Input: dimensioned drawing with shaded views. Units: mm. Origin: part minimum x, y, z. A direction names the side the tool comes from. Give positions to 0.01 mm unless a question says otherwise; leave off trailing zeros. Write each loop counter-clockwise with the first axis right and the second up, starting at its lowest first coordinate (ties: lowest second). Pieces come first, ordered by that corner, then holes. Notation, with made-up numbers: (75.5, 79) -> (102.5, 79) arc R27 ccw to (102.5, 104) -> close; hole circle Ø3 at (-15, 86.5). An arc over 180 degrees is marked (long way). Return JSON: item names as keys, results as strings. Group by question number.
Item 1: Section D-D, the plane y = 19. Return loops of the section in (x, z), then the cut area to 3 significant figures.
Item 2: Set-up query: the marked faces 1, 2 and 3. Return all of +Z, -Z, +X, -X, +Y, -Y with unobstructed straight access to the full face (end or side cutting, diameter ignored); none if empty.
Item 3: Line query: line 1 (Y direction, x = 6, z = 2.4); line 2 (Y direction, x = 5.25, z = 1.35) (1 decimal); line 3 (X direction, y = 6, z = 2.2). Output: solid intervals per line, ascending. Write a range as [from, to].
Item 4: Mould query, pull axis X, two halves, no side actions, for the marked faces 4, 5 and 6. Classes: released by +X, released by -X, zero draft, split by the parting line, or undercut.
Item 5: Section B-B, the plane z = 0.9. Count the separate pieces of the cut face and the enclosed holes in it, then the cut area to 3 significant figures.
Item 6: Pin query (flat end, axial travel): P1, Ø5, axis at x = 5, y = 6.5, coming from the +Z side; P2, Ø2, axis at x = 6, y = 25, coming from the +Z side; P3, Ø3, axis at x = 10, z = 0.5, coming from the +Y side (1 decimal). Return the tip coordinate at first contact, or that it passes through.
Item 7: Section A-A, the plane y = 6. Return loops of the section in (x, z).
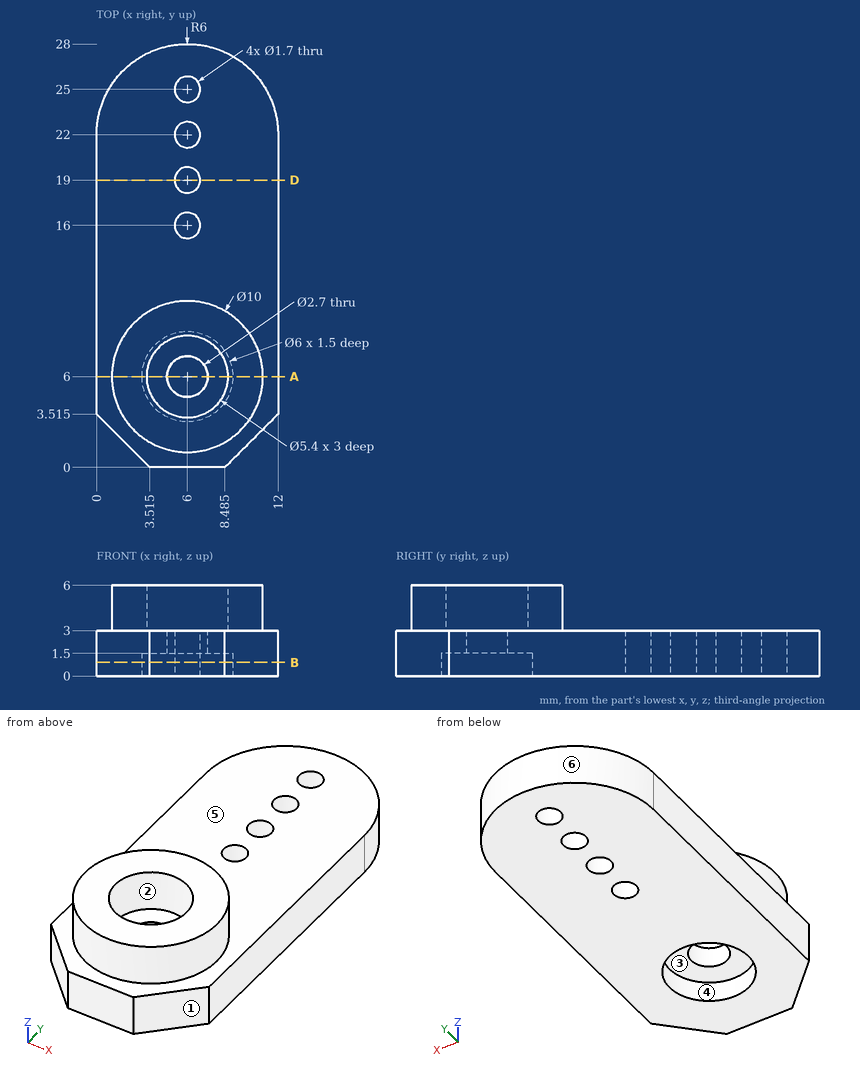
Answer below:
{
 "1": {"outline": "(0, 0) -> (5.15, 0) -> (5.15, 3) -> (0, 3) -> close; (6.85, 0) -> (12, 0) -> (12, 3) -> (6.85, 3) -> close", "area": "30.9 mm2"},
 "2": {"face 1": "+Z, -Z, +X, -Y", "face 2": "+Z", "face 3": "-Z"},
 "3": {"line 1": "y = [0, 4.65], [7.35, 15.15], [16.85, 18.15], [19.85, 21.15], [22.85, 24.15], [25.85, 28]", "line 2": "y = [0, 3.1], [8.9, 15.6], [16.4, 18.6], [19.4, 21.6], [22.4, 24.6], [25.4, 28]", "line 3": "x = [0, 4.65], [7.35, 12]"},
 "4": {"face 4": "undercut", "face 5": "zero draft", "face 6": "split by the parting line"},
 "5": {"separate pieces": "1", "enclosed holes": "5", "area": "271 mm2"},
 "6": {"P1": "stops at z = 6", "P2": "stops at z = 3", "P3": "stops at y = 27.5"},
 "7": {"outline": "(0, 0) -> (3, 0) -> (3, 1.5) -> (4.65, 1.5) -> (4.65, 3) -> (3.3, 3) -> (3.3, 6) -> (1, 6) -> (1, 3) -> (0, 3) -> close; (7.35, 1.5) -> (9, 1.5) -> (9, 0) -> (12, 0) -> (12, 3) -> (11, 3) -> (11, 6) -> (8.7, 6) -> (8.7, 3) -> (7.35, 3) -> close"}
}
